Print and shaded views of the part. All mm, measured from the part's lowest x, y and z. Round coordinates to 2 decimals unless told otherwise and drop trailing zeros. Loops run counter-clockwise (first coordinate to the right, second up) from the corner with the lowest first, then second, coordinate; pieces in that order, holes last. Notation, with made-up numbers: (-27.5, 21) -> (30.5, 21) arc R22 ccw to (30.5, 47) -> close; hole circle Ø4 at (57.25, 84). An arc over 180 degrees is marked (long way). Use a Markdown table: item, result.
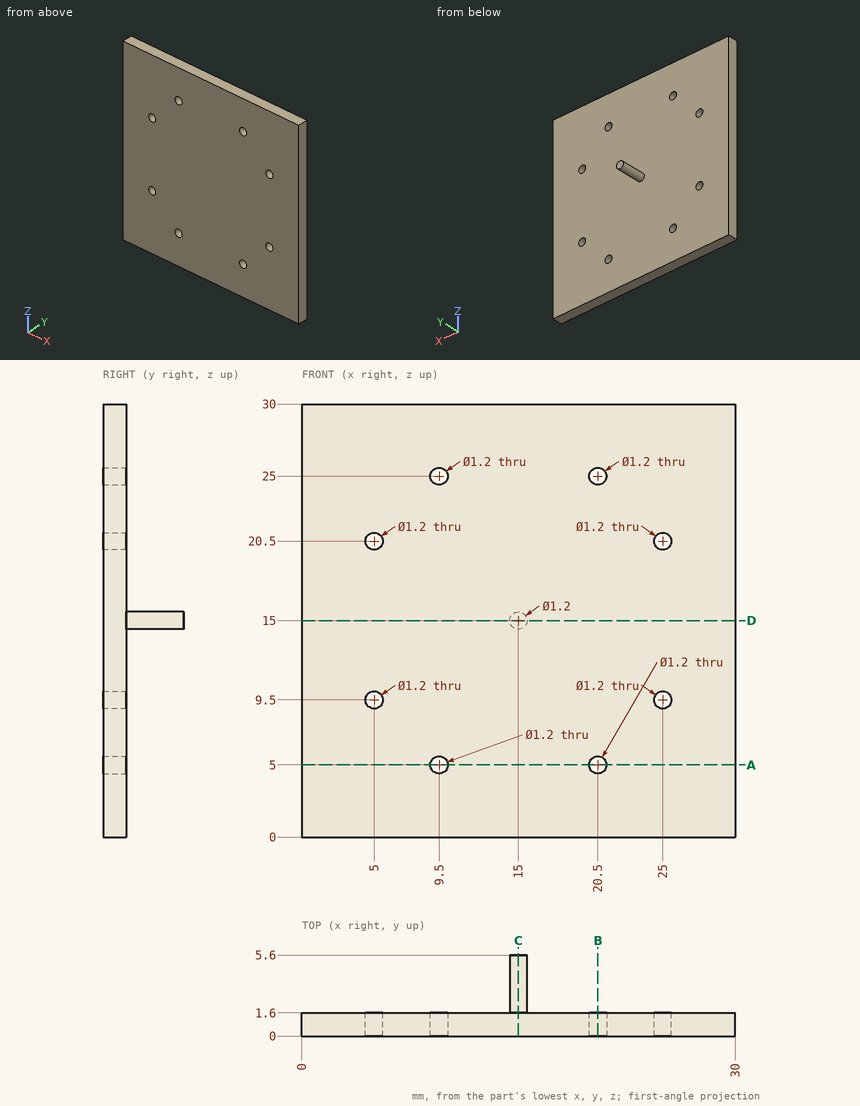
Q1. Band-saw the part on D-D, the plane z = 15. Give the cut face in (x, y), plus the area to 3 significant figures.
Results list:
| item | result |
|---|---|
| outline | (0, 0) -> (30, 0) -> (30, 1.6) -> (15.6, 1.6) -> (15.6, 5.6) -> (14.4, 5.6) -> (14.4, 1.6) -> (0, 1.6) -> close |
| area | 52.8 mm² |
Q2. Band-saw the part on B-B, the plane x = 20.5. Give the cut face in (y, z), plus the area to 3 significant figures.
Results list:
| item | result |
|---|---|
| outline | (0, 0) -> (1.6, 0) -> (1.6, 4.4) -> (0, 4.4) -> close; (0, 5.6) -> (1.6, 5.6) -> (1.6, 24.4) -> (0, 24.4) -> close; (0, 25.6) -> (1.6, 25.6) -> (1.6, 30) -> (0, 30) -> close |
| area | 44.2 mm² |
Q3. Flat gauge pin, fed straight in: pin 1 (1.6 mm diameter, centred on x = 20.5, z = 25, fed in from +Y). Where does the tip first touch, or does it go through?
Results list:
| item | result |
|---|---|
| pin 1 | stops at y = 1.6 |
Q4. Band-saw the part on A-A, the plane z = 5. Give the cut face in (x, y).
Results list:
| item | result |
|---|---|
| outline | (0, 0) -> (8.9, 0) -> (8.9, 1.6) -> (0, 1.6) -> close; (10.1, 0) -> (19.9, 0) -> (19.9, 1.6) -> (10.1, 1.6) -> close; (21.1, 0) -> (30, 0) -> (30, 1.6) -> (21.1, 1.6) -> close |
Q5. Drill centre lines: L1, parallel to X at y = 0.7, z = 5; L2, parallel to Z at x = 9.5, y = 0.6; L3, parallel to Z at x = 9.25, y = 0.65. Where is each one in solid material? Low to high. Write a range as from..to.
Results list:
| item | result |
|---|---|
| L1 | x = 0..8.9, 10.1..19.9, 21.1..30 |
| L2 | z = 0..4.4, 5.6..24.4, 25.6..30 |
| L3 | z = 0..4.45, 5.55..24.45, 25.55..30 |
Q6. Band-saw the part on C-C, the plane x = 15. Give the cut face in (y, z).
Results list:
| item | result |
|---|---|
| outline | (0, 0) -> (1.6, 0) -> (1.6, 14.4) -> (5.6, 14.4) -> (5.6, 15.6) -> (1.6, 15.6) -> (1.6, 30) -> (0, 30) -> close |
